Verification items for the finished model (mm, model axes). A direction names the side the tool comes from. Give positions to 0.01 mm unless a question says otherwise; leave off trailing zeros. Write each loop counter-clockwise with the first axis right and the second up, starting at its lowest first coordinate (ties: lowest second). Pieces come first, ordered by that corner, then holes.
from build123d import *

# Parameters (mm, degrees)
SKETCH1_R           = 4.4
BOSS_EXTRUDE1_DEPTH = 3
SKETCH2_R           = 1.6
BOSS_EXTRUDE2_DEPTH = 50
CUT_EXTRUDE1_DEPTH  = 10
CUT_EXTRUDE2_DEPTH  = 10


with BuildPart() as part:
    # Sketch1 → Boss-Extrude1 (new body)
    with BuildSketch(Plane.XY):
        with BuildLine():
            Line((-50, 45), (50, 45))
            ThreePointArc((50, 45), (57.071067812, 42.071067812), (60, 35))
            Line((60, 35), (60, -35))
            ThreePointArc((60, -35), (57.071067812, -42.071067812), (50, -45))
            Line((50, -45), (-50, -45))
            ThreePointArc((-50, -45), (-57.071067812, -42.071067812), (-60, -35))
            Line((-60, -35), (-60, 35))
            ThreePointArc((-60, 35), (-57.071067812, 42.071067812), (-50, 45))
        make_face()
        with Locations((0, 22.5)):
            Circle(SKETCH1_R, mode=Mode.SUBTRACT)
        with Locations((0, -22.5)):
            Circle(SKETCH1_R, mode=Mode.SUBTRACT)
    extrude(amount=BOSS_EXTRUDE1_DEPTH)

    # Sketch2 → Boss-Extrude2 (add)
    with BuildSketch(Plane(origin=(0, -44.902942235, 3), x_dir=(1, 0, 0), z_dir=(0, 0, 1))):
        with BuildLine():
            Line((-50, 0), (50, 0))
            ThreePointArc((50, 0), (57.071067812, 2.928932188), (60, 10))
            Line((60, 10), (60, 79.887698494))
            ThreePointArc((60, 79.887698494), (57.071067812, 86.958766306), (50, 89.887698494))
            Line((50, 89.887698494), (-50, 89.887698494))
            ThreePointArc((-50, 89.887698494), (-57.071067812, 86.958766306), (-60, 79.887698494))
            Line((-60, 79.887698494), (-60, 10))
            ThreePointArc((-60, 10), (-57.071067812, 2.928932188), (-50, 0))
        make_face()
        with Locations((-50, 79.887698494)):
            Circle(SKETCH2_R, mode=Mode.SUBTRACT)
        with Locations((-50, 10)):
            Circle(SKETCH2_R, mode=Mode.SUBTRACT)
        with Locations((50, 10)):
            Circle(SKETCH2_R, mode=Mode.SUBTRACT)
        with Locations((50, 79.887698494)):
            Circle(SKETCH2_R, mode=Mode.SUBTRACT)
        with BuildLine():
            Line((-45, 10), (-45, 3))
            Line((-45, 3), (45, 3))
            Line((45, 3), (45, 10))
            ThreePointArc((45, 10), (46.464466094, 13.535533906), (50, 15))
            Line((50, 15), (57, 15))
            Line((57, 15), (57, 74.887698494))
            Line((57, 74.887698494), (50, 74.887698494))
            ThreePointArc((50, 74.887698494), (46.464466094, 76.352164588), (45, 79.887698494))
            Line((45, 79.887698494), (45, 84.887698494))
            Line((45, 84.887698494), (-45, 84.887698494))
            Line((-45, 84.887698494), (-45, 79.887698494))
            ThreePointArc((-45, 79.887698494), (-46.464466094, 76.352164588), (-50, 74.887698494))
            Line((-50, 74.887698494), (-57, 74.887698494))
            Line((-57, 74.887698494), (-57, 15))
            Line((-57, 15), (-50, 15))
            ThreePointArc((-50, 15), (-46.464466094, 13.535533906), (-45, 10))
        make_face(mode=Mode.SUBTRACT)
    extrude(amount=BOSS_EXTRUDE2_DEPTH)

    # Sketch6 → Cut-Extrude1 (cut)
    with BuildSketch(Plane(origin=(0, 44.984756259, 0), x_dir=(1, 0, 0), z_dir=(0, 1, 0))):
        with BuildLine():
            Line((-4, -28), (-4, -53))
            Line((-4, -53), (4, -53))
            Line((4, -53), (4, -28))
            ThreePointArc((4, -28), (0, -24), (-4, -28))
        make_face()
    extrude(amount=-CUT_EXTRUDE1_DEPTH, mode=Mode.SUBTRACT)

    # Sketch7 → Cut-Extrude2 (cut)
    with BuildSketch(Plane.ZY.offset(60)):
        with BuildLine():
            Line((28, 4), (53, 4))
            Line((53, 4), (53, -4))
            Line((53, -4), (28, -4))
            ThreePointArc((28, -4), (24, 0), (28, 4))
        make_face()
    extrude(amount=-CUT_EXTRUDE2_DEPTH, mode=Mode.SUBTRACT)


solid = part.part
Item 1: Set-up check for faces 4 (the face through (56.993, -42.051, 27.65)), 5 (the face through (-59, 4, 40)), 6 (the face through (1, 1, 0)), 7 (the face through (-1, -41.903, 28)), 8 (the face through (-1, -44.903, 28)): record each of +Z, -Z, +X, -X, +Y, -Y from which the full face is reachable in a straight line by a thin tool's end or side.
Answer key:
face 4: +Z, +X, -Y
face 5: +Z, -X
face 6: -Z, +X, -X, +Y, -Y
face 7: +Z
face 8: +Z, +X, -X, -Y
Item 2: Release check for a two-part mould opening along X. For faces 1 (the face through (57.15, -41.99, 1.48)), 2 (the face through (46.426, -31.406, 27.65)), 3 (the face through (-59, 0, 24)) record: released by +X, released by -X, zero draft, split by the parting line, or undercut.
Answer key:
face 1: released by +X
face 2: undercut
face 3: zero draft
Item 3: Scan lines: line 1 along Y through (x, z) = (-41.5, 10.5); line 2 along X through (y, z) = (26, 22); line 3 along Y through (x, z) = (50, 18). Record each from-to range of solid material in increasing order.
Answer key:
line 1: y = -44.9 to -41.9, 39.98 to 44.98
line 2: x = -60 to -57, 57 to 60
line 3: y = -44.9 to -36.5, -33.3 to -29.9, 29.98 to 33.38, 36.58 to 44.98
Item 4: Sectioned sample at A-A on y = 22.5. Record the cut outline in (x, z), then the cut area to 3 significant figures.
Answer key:
outline: (-60, 0) - (-4.4, 0) - (-4.4, 3) - (-57, 3) - (-57, 53) - (-60, 53) - close; (4.4, 0) - (60, 0) - (60, 53) - (57, 53) - (57, 3) - (4.4, 3) - close
area: 634 mm2
Item 5: Depth check by flat-ended pin: pin 1 (1 mm diameter, centred on x = -12, z = 13.5, fed in from +Y); pin 2 (3.5 mm diameter, centred on x = -58, z = 34.5, fed in from +Y); pin 3 (14 mm diameter, centred on x = 0, y = -22.5, fed in from +Z). Enter the tip coordinate at first touch or a pass-through.
Answer key:
pin 1: stops at y = 44.98
pin 2: stops at y = 42.79
pin 3: stops at z = 3
Item 6: Sectioned sample at C-C on z = 5.5. Record the cut outline in (x, y), then the cut area to 3 significant figures.
Answer key:
outline: (-60, -34.9) arc R10 ccw to (-50, -44.9) - (50, -44.9) arc R10 ccw to (60, -34.9) - (60, 34.98) arc R10 ccw to (50, 44.98) - (-50, 44.98) arc R10 ccw to (-60, 34.98) - close; hole (-57, -29.9) - (-50, -29.9) arc R5 cw to (-45, -34.9) - (-45, -41.9) - (45, -41.9) - (45, -34.9) arc R5 cw to (50, -29.9) - (57, -29.9) - (57, 29.98) - (50, 29.98) arc R5 cw to (45, 34.98) - (45, 39.98) - (-45, 39.98) - (-45, 34.98) arc R5 cw to (-50, 29.98) - (-57, 29.98) - close; hole circle Ø3.2 at (-50, -34.9); hole circle Ø3.2 at (-50, 34.98); hole circle Ø3.2 at (50, -34.9); hole circle Ø3.2 at (50, 34.98)
area: 1,840 mm2
Item 7: Sectioned sample at D-D on y = -13.5. Record the cut outline in (x, z), then the cut area to 3 significant figures.
Answer key:
outline: (-60, 0) - (60, 0) - (60, 53) - (57, 53) - (57, 3) - (-57, 3) - (-57, 53) - (-60, 53) - close
area: 660 mm2
